```python
from build123d import *

# Parameters (mm, degrees)
F0_W        = 76.2
F0_H        = 38.1
F1_DEPTH    = 25.4
F2_R        = 6.35
F3_DEPTH    = 25.4
F4_R        = 12.7
F5_DEPTH    = 38.1
F6_W        = 12.7
F6_H        = 12.7
F8_T1_DEPTH = 101.6
F8_T3_DEPTH = 63.5


# Not quite as in the source:
# - a fillet or chamfer that OpenCascade refuses, or shapes differently, is made with other operations: its cross-section is extruded or revolved along the edge and cut away or added


with BuildPart() as f1:
    # F0 (on Top) → F1 (new body)
    with BuildSketch(Plane.XY):
        Rectangle(F0_W, F0_H)
    extrude(amount=F1_DEPTH)

    # F2 (on face) → F3 (cut)
    with BuildSketch(Plane.XY.offset(25.4)):
        with Locations((-30.48, 11.43)):
            Circle(F2_R)
        with Locations((-30.48, -11.43)):
            Circle(F2_R)
        with Locations((30.48, 11.43)):
            Circle(F2_R)
        with Locations((30.48, -11.43)):
            Circle(F2_R)
    extrude(amount=-F3_DEPTH, mode=Mode.SUBTRACT)

    # F4 (on face) → F5 (join)
    with BuildSketch(Plane.XY.offset(25.4)):
        Circle(F4_R)
    extrude(amount=F5_DEPTH)

    # F6 (on Front) → F7 (revolve, cut)
    with BuildSketch(Plane.XZ):
        with Locations((-10.1681923658, 47.7745333523)):
            Rectangle(F6_W, F6_H)
    revolve(axis=Axis((0, 0, 63.5), (0, 0, 1)), mode=Mode.SUBTRACT)

    # F8: fillet of radius 5.08 on 6 edges, made by hand

    # F8_s2 → F8_t1 (cut)
    with BuildSketch(Plane.YZ.offset(-50.8)):
        with BuildLine():
            ThreePointArc((-13.97, 25.4), (-17.5621024484, 23.9121024484), (-19.05, 20.32))
            Line((-19.05, 20.32), (-19.05, 25.4))
            Line((-19.05, 25.4), (-13.97, 25.4))
        make_face()
        with BuildLine():
            ThreePointArc((19.05, 20.32), (17.5621024484, 23.9121024484), (13.97, 25.4))
            Line((13.97, 25.4), (19.05, 25.4))
            Line((19.05, 25.4), (19.05, 20.32))
        make_face()
    extrude(amount=F8_T1_DEPTH, mode=Mode.SUBTRACT)

    # F8_s4 → F8_t3 (cut)
    with BuildSketch(Plane.XZ.offset(-31.75)):
        with BuildLine():
            ThreePointArc((-38.1, 20.32), (-36.6121024484, 23.9121024484), (-33.02, 25.4))
            Line((-33.02, 25.4), (-38.1, 25.4))
            Line((-38.1, 25.4), (-38.1, 20.32))
        make_face()
        with BuildLine():
            ThreePointArc((38.1, 20.32), (36.6121024484, 23.9121024484), (33.02, 25.4))
            Line((33.02, 25.4), (38.1, 25.4))
            Line((38.1, 25.4), (38.1, 20.32))
        make_face()
    extrude(amount=F8_T3_DEPTH, mode=Mode.SUBTRACT)

    # F8_s5 → F8_t6 (revolve, cut)
    with BuildSketch(Plane.XZ):
        with BuildLine():
            ThreePointArc((12.7, 36.3445333523), (11.2121024484, 39.9366358007), (7.62, 41.4245333523))
            Line((7.62, 41.4245333523), (12.7, 41.4245333523))
            Line((12.7, 41.4245333523), (12.7, 36.3445333523))
        make_face()
    revolve(axis=Axis((0, 0, 41.4245333523), (0, 0, -1)), mode=Mode.SUBTRACT)

    # F8_s7 → F8_t8 (revolve, cut)
    with BuildSketch(Plane.XZ):
        with BuildLine():
            ThreePointArc((7.62, 54.1245333523), (11.2121024484, 55.6124309038), (12.7, 59.2045333523))
            Line((12.7, 59.2045333523), (12.7, 54.1245333523))
            Line((12.7, 54.1245333523), (7.62, 54.1245333523))
        make_face()
    revolve(axis=Axis((0, 0, 54.1245333523), (0, 0, -1)), mode=Mode.SUBTRACT)

    # F9: chamfer of 5.08 on 1 edges, made by hand

    # F9_s1 → F9_t2 (revolve, cut)
    with BuildSketch(Plane.XZ):
        Polygon((12.7, 58.42), (7.62, 63.5), (12.7, 63.5), align=None)
    revolve(axis=Axis((0, 0, 63.5), (0, 0, 1)), mode=Mode.SUBTRACT)


solid = f1.part
```
Read the model definition and answer for the solid it produces. Units are mm, in the model's axes. A direction names the side the tool comes from. Coordinates: 2 decimals unless noted, no trailing zeros. Write each loop counter-clockwise with the first axis right and the second up, starting at its lowest first coordinate (ties: lowest second). Pieces come first, ordered by that corner, then holes. Notation, with made-up numbers: (28.25, 82) -> (41.25, 82) arc R26 cw to (41.25, 110) -> close; hole circle Ø6 at (-33.75, -33). An arc over 180 degrees is marked (long way). Write item = value, one per line.
(1) Section D-D on y = -11.43 is taken. Count the separate pieces of the cut face and the enclosed holes in it, plus the area to 3 significant figures.
From the geometry:
separate_pieces = 4
enclosed_holes = 0
area = 1,460 mm2
(2) Which of the six approach directions +Z, -Z, +X, -X, +Y, -Y give full straight-line access (tool end or side, diameter ignored) to faces 1 (the face through (-2.75, -12.4, 30.8)), 2 (the face through (-1, 0, 0)), 3 (the face through (-3, 3, 41.425))?
From the geometry:
face_1 = +Z
face_2 = -Z, +X, -X, +Y, -Y
face_3 = none
(3) Given pin 1 Ø8 at (y, z) = (7.5, 48) entering from +X; pin 2 Ø7.5 at (x, y) = (-30.48, 11.43) entering from +Z; pin 3 Ø10 at (x, y) = (11.5, 13) entering from -Z; pin 4 Ø8 at (x, z) = (-1.5, 45.5) entering from +Y, each flat-ended and moving along its own axis, determine where each tip first touches the part or whether it passes through.
From the geometry:
pin_1 = 1.53
pin_2 = through
pin_3 = 0
pin_4 = 3.82
(4) Section A-A on x = 0 is taken. Write down the section's boundary in (y, z), plus the area to 3 significant figures.
From the geometry:
outline = (-19.05, 0) -> (19.05, 0) -> (19.05, 20.32) arc R5.08 ccw to (13.97, 25.4) -> (12.7, 25.4) -> (12.7, 36.34) arc R5.08 ccw to (7.62, 41.42) -> (3.82, 41.42) -> (3.82, 54.12) -> (7.62, 54.12) arc R5.08 ccw to (12.65, 58.47) -> (7.62, 63.5) -> (-7.62, 63.5) -> (-12.65, 58.47) arc R5.08 ccw to (-7.62, 54.12) -> (-3.82, 54.12) -> (-3.82, 41.42) -> (-7.62, 41.42) arc R5.08 ccw to (-12.7, 36.34) -> (-12.7, 25.4) -> (-13.97, 25.4) arc R5.08 ccw to (-19.05, 20.32) -> close
area = 1,650 mm2
(5) Section C-C on y = 0 is taken. Write down the section's boundary in (x, z), plus the area to 3 significant figures.
From the geometry:
outline = (-38.1, 0) -> (38.1, 0) -> (38.1, 20.32) arc R5.08 ccw to (33.02, 25.4) -> (12.7, 25.4) -> (12.7, 36.34) arc R5.08 ccw to (7.62, 41.42) -> (3.82, 41.42) -> (3.82, 54.12) -> (7.62, 54.12) arc R5.08 ccw to (12.65, 58.47) -> (7.62, 63.5) -> (-7.62, 63.5) -> (-12.65, 58.47) arc R5.08 ccw to (-7.62, 54.12) -> (-3.82, 54.12) -> (-3.82, 41.42) -> (-7.62, 41.42) arc R5.08 ccw to (-12.7, 36.34) -> (-12.7, 25.4) -> (-33.02, 25.4) arc R5.08 ccw to (-38.1, 20.32) -> close
area = 2,620 mm2
(6) Straight lines are drawn through the part: L1, parallel to X at y = 11.43, z = 5; L2, parallel to Y at x = -30.48, z = 8; L3, parallel to Y at x = 32, z = 4.5. For each, find the intervals that lie inside material, in ascending order. Write a range as from..to.
From the geometry:
L1 = -38.1..-36.83, -24.13..24.13, 36.83..38.1
L2 = -19.05..-17.78, -5.08..5.08, 17.78..19.05
L3 = -19.05..-17.6, -5.26..5.26, 17.6..19.05
(7) For a pull along Y with two mould halves and no side action, classify faces 4 (the face through (-38.1, 0, 10)), 5 (the face through (25.44, 7.57, 12.88)), 6 (the face through (-2.05, -3.22, 47.86)) as +Y half, -Y half, draft (parallel to the pull), parting line (faces both ways), or undercut.
From the geometry:
face_4 = draft
face_5 = undercut
face_6 = parting line
(8) Section B-B on x = 30.48 is taken. Write down the section's boundary in (y, z).
From the geometry:
outline = (-19.05, 0) -> (-17.78, 0) -> (-17.78, 23.68) arc R5.08 ccw to (-19.05, 20.32) -> close; (-5.08, 0) -> (5.08, 0) -> (5.08, 25.4) -> (-5.08, 25.4) -> close; (17.78, 0) -> (19.05, 0) -> (19.05, 20.32) arc R5.08 ccw to (17.78, 23.68) -> close
